For this review, take the finished solid that the model builds, in its own axes (mm). A direction names the side the tool comes from. Coordinates: 2 decimals unless noted, no trailing zeros. Write each loop counter-clockwise with the first axis right and the second up, starting at its lowest first coordinate (ties: lowest second). Pieces come first, ordered by that corner, then holes. Notation, with made-up numbers: (51, 52) - (57, 52) arc R25 cw to (57, 65) - close; hole circle Ø4 at (58, 89.25). An arc over 180 degrees is marked (long way). Write each question's results on one line, items separated by ' | '.
Autodesk Inventor part; units mm, degrees
ref_plane "YZ Plane" through (0, 0, 0) normal (1, 0, 0) x (0, 1, 0)
ref_plane "XZ Plane" through (0, 0, 0) normal (0, 1, 0) x (-1, 0, 0)
ref_plane "XY Plane" through (0, 0, 0) normal (0, 0, 1) x (1, 0, 0)
sketch "Szkic1" plane through (0, 0, 0) normal (0, 1, 0) x (-1, 0, 0)
  circle A0 centre (0, 0) radius 50
  circle A1 centre (0, 0) radius 45
  line L0 (-5.5, 26) -> (5.5, 26)
  line L1 (5.5, 26) -> (5.5, 16)
  line L2 (5.5, 16) -> (-5.5, 16)
  line L3 (-5.5, 16) -> (-5.5, 26)
  line L4 (-5.5, 26) -> (5.5, 16) construction
  line L5 (5.5, 26) -> (-5.5, 16) construction
  line L6 (-5.5, -6.25) -> (5.5, -6.25)
  line L7 (5.5, -6.25) -> (5.5, -16.25)
  line L8 (5.5, -16.25) -> (-5.5, -16.25)
  line L9 (-5.5, -16.25) -> (-5.5, -6.25)
  line L10 (-5.5, -6.25) -> (5.5, -16.25) construction
  line L11 (5.5, -6.25) -> (-5.5, -16.25) construction
  point P0 (0, 21)
  point P1 (0, -11.25)
  point P2 (0, 16)
  dimension "d0" = 100
  dimension "d1" = 90
  dimension "d2" = 11
  dimension "d3" = 10
  dimension "d4" = 11
  dimension "d5" = 10
  dimension "d6" = 6.25
  dimension "d7" = 16
extrude "Wyciągnięcie proste1" add sketch "Szkic1" along normal blind 25 contours L0 L1 L2 L3 | L6 L7 L8 L9
extrude "Wyciągnięcie proste2" add sketch "Szkic1" along normal blind 38 contours A0
extrude "Wyciągnięcie proste3" add sketch "Szkic1" along normal blind 4 contours A1
sketch "Szkic2" plane through (5.5, 25, 26) normal (1, 0, 0) x (0, 0, -1)
  line L0 (10, -21) -> (10, 0)
  line L1 (10, -10.5) -> (4, -10.5)
  line L2 (4, -10.5) -> (4, -20.5)
  line L3 (4, -20.5) -> (10, -20.5)
  line L4 (10, -20.5) -> (10, -10.5)
  line L5 (32.25, -21) -> (32.25, 0)
  line L6 (32.25, -10.5) -> (38.25, -10.5)
  line L7 (38.25, -10.5) -> (38.25, -20.5)
  line L8 (38.25, -20.5) -> (32.25, -20.5)
  line L9 (32.25, -20.5) -> (32.25, -10.5)
  point P0 (26, -25)
  point P1 (10, -20.5)
  dimension "d14" = 6
  dimension "d15" = 10
  dimension "d16" = 6
  dimension "d17" = 10
extrude "Wyciągnięcie proste4" cut sketch "Szkic2" against normal blind 11
ref_plane "Płaszczyzna konstrukcyjna1" through (0, 25, 16) normal (-1, 0, 0) x (0, 0, 1)
sketch "Szkic3" plane through (0, 25, 16) normal (-1, 0, 0) x (0, 0, 1)
  circle A0 centre (-11.25, -10.5) radius 6
  point P0 (-16, -25)
  dimension "d20" = 12
extrude "Wyciągnięcie proste5" cut sketch "Szkic3" against normal through all
sketch "Szkic4" plane through (0, 0, 0) normal (0, -1, 0) x (1, 0, 0)
  point P0 (0, 0)
properties part number "podstawa roobota_Drukowanie 3D"
Q1. Wall thickness on line 1 along Z through (x, y) = (0, 22); line 2 along Y through (x, z) = (46, 4.75); line 3 along Y through (x, z) = (-32, -19): over which ranges is each line inside the solid? List them lowest first. Write a range as from..to.
Results found:
line 1: -50..-45, -16.25..-6.25, 16..26, 45..50 | line 2: 0..8.5, 20.5..38 | line 3: 0..4
Q2. Take a section at A-A on z = 5. State the section outline as (x, y) points, plus the area to 3 significant figures.
Results found:
outline: (-49.75, 0) - (49.75, 0) - (49.75, 8.51) - (44.72, 8.51) - (44.72, 4) - (-44.72, 4) - (-44.72, 38) - (-49.75, 38) - close; (44.72, 20.49) - (49.75, 20.49) - (49.75, 38) - (44.72, 38) - close | area: 680 mm2
Q3. Take a section at D-D on z = -28. State the section outline as (x, y) points.
Results found:
outline: (-41.42, 0) - (41.42, 0) - (41.42, 38) - (35.23, 38) - (35.23, 4) - (-35.23, 4) - (-35.23, 38) - (-41.42, 38) - close
Q4. Take a section at B-B on x = 0. State the section outline as (y, z) points.
Results found:
outline: (0, -50) - (38, -50) - (38, -45) - (4, -45) - (4, -16.25) - (25, -16.25) - (25, -6.25) - (14.5, -6.25) - (14.5, -12.25) - (4.5, -12.25) - (4.5, -6.25) - (4, -6.25) - (4, 16) - (4.5, 16) - (4.5, 22) - (14.5, 22) - (14.5, 16) - (25, 16) - (25, 26) - (4, 26) - (4, 45) - (38, 45) - (38, 50) - (0, 50) - close
Q5. Take a section at C-C on y = 28. State the section outline as (x, z) points.
Results found:
outline: circle Ø100 at (0, 0); hole circle Ø90 at (0, 0)
Q6. For faces 1 (the face through (5.5, 17, -12)), 2 (the face through (-47.69, 18.73, -15.02)), 3 (the face through (0, 10, -12.25)), list the 3-axis set-ups (+Z, -Z, +X, -X, +Y, -Y) from which the entire face can be reached by the end or side of a thin tool; tool diameter is ignored.
Results found:
face 1: +Y | face 2: +Y, -Y | face 3: none
Q7. For pin 1 (8 mm diameter, centred on x = 0.5, z = 19.5, fed in from +Y); pin 2 (8 mm diameter, centred on x = -21.5, y = 5.5, fed in from -Z); pin 3 (11.5 mm diameter, centred on x = 0, y = 20, fed in from -Z), all flat-tipped, find the tip position at first contact; note any pin that passes through.
Results found:
pin 1: y = 25 | pin 2: z = -46.84 | pin 3: z = -50
Q8. Mouldability with a two-part tool opening along Y and no side actions: class faces 4 (the face through (1, 0, 1)), 5 (the face through (0, 20, -6.25)), 6 (the face through (0, 25, 21)), 7 (the face through (46.8, 12.2, 10.29)) as pulls with the +Y half, pulls with the -Y half, needs draft (parallel to the pull), parting line crosses it, or undercut.
Results found:
face 4: pulls with the -Y half | face 5: needs draft | face 6: pulls with the +Y half | face 7: undercut
